Could you check a few things on this model? Use its own coordinates, in mm. Give positions to 0.01 mm unless a question says otherwise; leave off trailing zeros. Order: outer loops, then holes, each group sorted by start corner. A loop starts at its lowest first (then second) coordinate and runs counter-clockwise, first axis right, second up. Notation, with made-up numbers: M 60.25,74 L 71.25,74 A21 cw 71.25,87 Z; hole C -23,71 d4. An arc over 180 degrees is marked long. Use a Markdown table: item, result. Add a question column.
Autodesk Inventor part; units mm, degrees
ref_plane "YZ Plane" through (0, 0, 0) normal (1, 0, 0) x (0, 1, 0)
ref_plane "XZ Plane" through (0, 0, 0) normal (0, 1, 0) x (-1, 0, 0)
ref_plane "XY Plane" through (0, 0, 0) normal (0, 0, 1) x (1, 0, 0)
sketch "Sketch1" plane through (0, 0, 0) normal (0, 1, 0) x (-1, 0, 0)
  line L0 (374.9202, -60.2574) -> (324.1202, -60.2574)
  line L1 (324.1202, -60.2574) -> (324.1202, -263.4574)
  line L2 (324.1202, -263.4574) -> (374.9202, -263.4574)
  line L3 (374.9202, -263.4574) -> (374.9202, -60.2574)
  point P0 (0, 0)
  dimension "d0" = 203.2
  dimension "d1" = 50.8
extrude "Extrusion1" add sketch "Sketch1" along normal blind 2.9972
sketch "Sketch2" plane through (0, 2.9972, 0) normal (0, 1, 0) x (1, 0, 0)
  line L0 (-336.8202, 206.3074) -> (-362.2202, 206.3074) construction
  line L1 (-362.2202, 206.3074) -> (-362.2202, 250.7574) construction
  line L2 (-362.2202, 250.7574) -> (-336.8202, 250.7574) construction
  line L3 (-336.8202, 250.7574) -> (-336.8202, 206.3074) construction
  line L4 (-336.8202, 206.3074) -> (-362.2202, 250.7574) construction
  line L5 (-362.2202, 206.3074) -> (-336.8202, 250.7574) construction
  line L6 (-324.1202, 263.4574) -> (-374.9202, 263.4574)
  line L7 (-349.5202, 228.5324) -> (-349.5202, 263.4574) construction
  circle A0 centre (-362.2202, 250.7574) radius 2.1828
  circle A1 centre (-336.8202, 250.7574) radius 2.1828
  circle A2 centre (-336.8202, 206.3074) radius 2.1828
  circle A3 centre (-362.2202, 206.3074) radius 2.1828
  point P0 (0, 0)
  dimension "d4" = 25.4
  dimension "d5" = 44.45
  dimension "d6" = 12.7
  dimension "d7" = 4.3656
extrude "Extrusion2" cut sketch "Sketch2" against normal through all
properties part number "8x2 Lexan" material "Polycarbonate, Clear"
1) We'd pull the mould along Z, two halves only. Please class faces 1 (the face through (-349, 2.997, -160)), 2 (the face through (-360.138, 1.52, -251.413)): pulls with the +Z half, pulls with the -Z half, needs draft (parallel to the pull), parting line crosses it, or undercut.
2) Suppose I cut it at A-A on x = -336.5. Please give me the cut outline in (y, z), and give its area (3 significant figures).
3) Please list where these lines run through material, in increasing order: line 1 (X direction, y = 1.3, z = -205); line 2 (Z direction, x = -336, y = 2.4). Write a range as from..to.
4) For pin 1 (7 mm diameter, centred on x = -336.82, z = -206.31, fed in from +Y), with a flat end and sliding along its axis, tell me the tip position at first contact or that it passes through.
Values found:
| question | item | result |
|---|---|---|
| 1 | face 1 | needs draft |
| 1 | face 2 | undercut |
| 2 | outline | M 0,-263.46 L 3,-263.46 L 3,-252.92 L 0,-252.92 Z; M 0,-248.6 L 3,-248.6 L 3,-208.47 L 0,-208.47 Z; M 0,-204.15 L 3,-204.15 L 3,-60.26 L 0,-60.26 Z |
| 2 | area | 583 mm^2 |
| 3 | line 1 | x = -374.92..-363.97, -360.47..-338.57, -335.07..-324.12 |
| 3 | line 2 | z = -263.46..-252.78, -248.73..-208.33, -204.28..-60.26 |
| 4 | pin 1 | stops at y = 3 |
